from build123d import *

# Parameters (mm, degrees)
PAD_DEPTH    = 0.5
SKETCH001_R  = 0.25
PAD001_DEPTH = 0.01


with BuildPart() as part:
    # Sketch (on YZ_Plane of Origin) → Pad (new body)
    with BuildSketch(Plane.YZ):
        Polygon((-4.5, -5.5), (4.5, -5.5), (4.5, 5), (4, 5.5), (-4.5, 5.5), align=None)
    extrude(amount=PAD_DEPTH)

    # Sketch001 (on Face7 of Pad) → Pad001 (join)
    with BuildSketch(Plane.YZ.offset(0.5)):
        with Locations((-3.5, 4.5)):
            Circle(SKETCH001_R)
    extrude(amount=PAD001_DEPTH)


solid = part.part
Design review of the part built by this model. Coordinates are the model's own, in mm. Round coordinates to 2 decimals unless told otherwise and drop trailing zeros. Write each loop counter-clockwise with the first axis right and the second up, starting at its lowest first coordinate (ties: lowest second). Pieces come first, ordered by that corner, then holes. Notation, with made-up numbers: (-16.75, 7.5) - (34.25, 7.5) arc R16 ccw to (34.25, 26.5) - close; hole circle Ø4 at (20.5, 45.25). An arc over 180 degrees is marked (long way). Return JSON: item names as keys, results as strings. Group by question number.
Item 1: We need section D-D on z = 1.25. Write out the cut boundary in (x, y).
Item 2: For probe 1 along X at (y, z) = (-3.25, -3.75); probe 2 along Y at (x, z) = (0.3, 5.25), list the stretches that pass through material, from the lowest coordinate up. Write a range as [from, to].
Item 3: Insertion check: P1, Ø5, axis at y = 2.5, z = -1, coming from the +X side. The pin has a flat end and moves straight along its axis. Give the tip position at first contact, or say it passes through.
Item 4: We need section C-C on y = 0. Write out the cut boundary in (x, z).
Model answer:
{
 "1": {"outline": "(0, -4.5) - (0.5, -4.5) - (0.5, 4.5) - (0, 4.5) - close"},
 "2": {"probe 1": "x = [0, 0.5]", "probe 2": "y = [-4.5, 4.25]"},
 "3": {"P1": "stops at x = 0.5"},
 "4": {"outline": "(0, -5.5) - (0.5, -5.5) - (0.5, 5.5) - (0, 5.5) - close"}
}
